Geometry: final body of the model. Coordinates: model frame, mm. Face numbers are marked on the shaded views. A direction names the side the tool comes from. Round coordinates to 2 decimals unless told otherwise and drop trailing zeros. Loops run counter-clockwise (first coordinate to the right, second up) from the corner with the lowest first, then second, coordinate; pieces in that order, holes last. Notation, with made-up numbers: (63, -36) - (76, -36) arc R26 cw to (76, -18) - close; hole circle Ø8 at (1, -21.5). An arc over 180 degrees is marked (long way). Answer as a JSON object with one key per item and string values. Group by question number.
Item 1: Section A-A (z = 0). Return the cut outline in (x, y) (3 decimals), plus the area to 3 significant figures.
Item 2: Line query: line 1 (Z direction, x = 2.75, y = 0) (3 decimals); line 2 (Y direction, x = 2.5, z = 0) (3 decimals); line 3 (X direction, y = 5.5, z = 2) (3 decimals). Output: solid intervals per line, ascending.
Item 3: Draft query along Y for the marked faces 4, 5, 6 and 7. Return one class per face: released by +Y, released by -Y, zero draft, split by the parting line, or undercut.
Item 4: Section B-B (x = 0). Return the cut outline in (y, z) (3 decimals), plus the area to 3 significant figures.
Item 5: Reachability of the marked faces 1, 2 and 3 from +Z, -Z, +X, -X, +Y, -Y: full face, straight path, thin tool, end or side. Return the list, or none.
Item 6: First-contact query: pin 1 (1.5 mm diameter, centred on x = -1, z = 6, fed in from +Y); pin 2 (1.5 mm diameter, centred on x = 1, y = -5.5, fed in from +Z); pin 3 (5 mm diameter, centred on y = -0.5, z = 2, fed in from +X). Flat tips, straight axial feed; report the tip coordinate or a pass-through.
Item 7: Section D-D (y = 14). Return the cut outline in (x, z), plus the area to 3 significant figures.
Item 8: Section C-C (x = 8.25). Return the cut outline in (y, z).
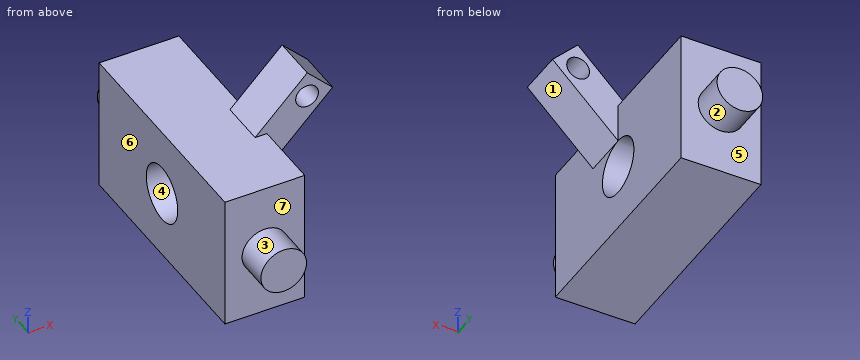
```python
from build123d import *

# Parameters (mm, degrees)
SKETCH1_W                = 8.89
SKETCH1_H                = 14.999999972
BOSS_EXTRUDE1_DEPTH      = 16.51
BOSS_EXTRUDE1_DEPTH_BACK = 16.51
SKETCH1_3_R              = 1.27
BOSS_EXTRUDE2_DEPTH      = 5.08
SKETCH3_W                = 16.776229269
SKETCH3_H                = 3.81
SKETCH4_R                = 3.175
CUT_EXTRUDE1_DEPTH       = 12.76066318
CUT_EXTRUDE1_DEPTH_BACK  = 5.445


with BuildPart() as part:
    # Sketch1 → Boss-Extrude1 (new body, two sides)
    with BuildSketch(Plane(origin=(0, 0, 0), x_dir=(1, 0, 0), z_dir=(0, 1, 0))) as boss_extrude1_sk:
        Rectangle(SKETCH1_W, SKETCH1_H)
    extrude(amount=BOSS_EXTRUDE1_DEPTH)
    extrude(boss_extrude1_sk.sketch, amount=-BOSS_EXTRUDE1_DEPTH_BACK)

    # Sketch1_3 → Boss-Extrude2 (add)
    with BuildSketch(Plane(origin=(0, 0, 0), x_dir=(1, 0, 0), z_dir=(0, 1, 0))):
        Polygon((11.76066318, -10.480507782), (4.445, -3.164844602), (4.445, -7.499999986), (3.123301134, -7.499999986), (8.932236056, -13.308934907), align=None)
        with Locations((8.909608639, -10.457880365)):
            Circle(SKETCH1_3_R, mode=Mode.SUBTRACT)
    extrude(amount=-BOSS_EXTRUDE2_DEPTH)

    # Sketch3 → Cut-Revolve1 (revolve, cut)
    with BuildSketch(Plane(origin=(0, 0, 0), x_dir=(0, 0, -1), z_dir=(1, 0, 0))):
        with Locations((-10.928114634, 14.605)):
            Rectangle(SKETCH3_W, SKETCH3_H)
        with Locations((-10.928114634, -14.605)):
            Rectangle(SKETCH3_W, SKETCH3_H)
    revolve(axis=Axis((0, 0, 0), (0, 1, 0)), mode=Mode.SUBTRACT)

    # Sketch4 → Cut-Extrude1 (cut, two sides)
    with BuildSketch(Plane(origin=(0, 0, 0), x_dir=(0, 0, -1), z_dir=(1, 0, 0))) as cut_extrude1_sk:
        Circle(SKETCH4_R)
    extrude(amount=CUT_EXTRUDE1_DEPTH, mode=Mode.SUBTRACT)
    extrude(cut_extrude1_sk.sketch, amount=-CUT_EXTRUDE1_DEPTH_BACK, mode=Mode.SUBTRACT)


solid = part.part
```
Values:
{
 "1": {"outline": "(-4.445, -12.7) - (-2.54, -12.7) - (-2.54, -16.51) - (2.54, -16.51) - (2.54, -12.7) - (4.445, -12.7) - (4.445, -3.175) - (-4.445, -3.175) - close; (-4.445, 3.175) - (4.445, 3.175) - (4.445, 12.7) - (2.54, 12.7) - (2.54, 16.51) - (-2.54, 16.51) - (-2.54, 12.7) - (-4.445, 12.7) - close", "area": "208 mm^2"},
 "2": {"line 1": "z = -7.5 to -3.175, 3.175 to 7.5", "line 2": "y = -16.51 to -3.175, 3.175 to 16.51", "line 3": "x = -4.445 to 4.445"},
 "3": {"face 4": "undercut", "face 5": "released by +Y", "face 6": "zero draft", "face 7": "released by -Y"},
 "4": {"outline": "(-16.51, -2.54) - (-12.7, -2.54) - (-12.7, -7.5) - (12.7, -7.5) - (12.7, -2.54) - (16.51, -2.54) - (16.51, 2.54) - (12.7, 2.54) - (12.7, 7.5) - (-12.7, 7.5) - (-12.7, 2.54) - (-16.51, 2.54) - close; hole circle Ø6.35 at (0, 0)", "area": "388 mm^2"},
 "5": {"face 1": "-Z, +X, +Y, -Y", "face 2": "+Y", "face 3": "-Y"},
 "6": {"pin 1": "stops at y = 12.7", "pin 2": "stops at z = 7.5", "pin 3": "stops at x = 5.78"},
 "7": {"outline": "circle Ø5.08 at (0, 0)", "area": "20.3 mm^2"},
 "8": {"outline": "(-5.08, 6.97) - (0, 6.97) - (0, 9.37) - (-5.08, 9.37) - close; (-5.08, 11.54) - (0, 11.54) - (0, 12.63) - (-5.08, 12.63) - close"}
}
